Input: part model. Units: mm. Frame: model coordinates. A direction names the side the tool comes from. Coordinates: 2 decimals unless noted, no trailing zeros. Loops run counter-clockwise (first coordinate to the right, second up) from the corner with the lowest first, then second, coordinate; pieces in that order, holes last.
```python
from build123d import *

# Parameters (mm, degrees)
EXTRUDE_1_DEPTH      = 2.5
EXTRUDE_1_DEPTH_BACK = 2.5
SKETCH_2_OUTSIDE_W   = 45.04
SKETCH_2_OUTSIDE_H   = 51.807
SKETCH_2_OUTSIDE_R   = 2
CUT_EXTRUDE_1_DEPTH  = 2.5
CUT_EXTRUDE_1_DRAFT  = -60
FILLET_2_R           = 4
FILLET_3_R           = 9
SKETCH_3_R           = 2
EXTRUDE_2_DEPTH      = 9
SKETCH_4_W           = 26.934408862
SKETCH_4_H           = 1.5
CUT_EXTRUDE_2_DEPTH  = 7
FILLET_4_R           = 0.5


with BuildPart() as part:
    # 草图1 → 凸台-拉伸1 (new, two sides: drawn at the far end of the back side and taken through both)
    with BuildSketch(Plane.XY.offset(-EXTRUDE_1_DEPTH_BACK)):
        Polygon((-1.165769145, -2.5), (-8.342987205, 6.053475407), (-4.512764989, 9.267413455), (1.165769145, 2.5), (138, 2.5), (138, -2.5), align=None)
    extrude(amount=EXTRUDE_1_DEPTH + EXTRUDE_1_DEPTH_BACK)


with BuildPart() as cut_extrude_1_tool:
    # 草图2 outside → 切除-拉伸1 (with draft: the straight prism first)
    with BuildSketch(Plane(origin=(138, 0, 0), x_dir=(0, 0, -1), z_dir=(1, 0, 0))):
        with Locations((0, 3.3835)):
            Rectangle(SKETCH_2_OUTSIDE_W, SKETCH_2_OUTSIDE_H)
        Circle(SKETCH_2_OUTSIDE_R, mode=Mode.SUBTRACT)
    extrude(amount=-CUT_EXTRUDE_1_DEPTH)
    # 切除-拉伸1: the draft: its side faces are tilted about the plane it starts from
    cut_extrude_1_sides = [cut_extrude_1_tool.faces().sort_by_distance(p)[0] for p in [
        (136.75, -22.52, 0),
        (136.75, 3.3835, -22.52),
        (136.75, 29.287, 0),
        (136.75, 3.3835, 22.52),
        (136.75, 0, 2),
    ]]
    draft(cut_extrude_1_sides, Plane(origin=(138, 0, 0), x_dir=(0, 0, -1), z_dir=(1, 0, 0)), CUT_EXTRUDE_1_DRAFT)


with BuildPart() as part_1:
    add(part.part)

    # 切除-拉伸1: cut by cut_extrude_1_tool
    add(cut_extrude_1_tool.part, mode=Mode.SUBTRACT)

    # 圆角2
    fillet_2_edges = [part_1.edges().sort_by_distance(p)[0] for p in [
        (1.165769145, 2.5, 0),
    ]]
    fillet(fillet_2_edges, radius=FILLET_2_R)

    # 圆角3
    fillet_3_edges = [part_1.edges().sort_by_distance(p)[0] for p in [
        (-1.165769145, -2.5, 0),
    ]]
    fillet(fillet_3_edges, radius=FILLET_3_R)

    # 草图3 → 凸台-拉伸2 (add)
    with BuildSketch(Plane(origin=(-6.427876097, 7.660444431, 0), x_dir=(0.7660444431189749, 0.6427876096865432, 0), z_dir=(-0.6427876096865431, 0.7660444431189748, 0))):
        Circle(SKETCH_3_R)
    extrude(amount=EXTRUDE_2_DEPTH)

    # 草图4 → 切除-拉伸2 (cut)
    with BuildSketch(Plane(origin=(-12.212964584, 14.554844419, 0), x_dir=(0.7660444431189747, 0.6427876096865435, 0), z_dir=(-0.6427876096865434, 0.7660444431189746, 0))):
        Rectangle(SKETCH_4_W, SKETCH_4_H)
    extrude(amount=-CUT_EXTRUDE_2_DEPTH, mode=Mode.SUBTRACT)

    # 圆角4
    fillet_4_edges = [part_1.edges().sort_by_distance(p)[0] for p in [
        (-7.959964983, 6.374869212, 0),
    ]]
    fillet(fillet_4_edges, radius=FILLET_4_R - 0.0001)  # a hair under: the kernel refuses the full size


solid = part_1.part
```
Item 1: Contact query for flat-ended pins moving along their axis: P1, Ø2, axis at x = -9, y = 12.5, coming from the -Z side; P2, Ø8, axis at x = -9.5, y = 11, coming from the +Z side. Output: stop coordinate, or through.
Result:
P1: stops at z = -2
P2: stops at z = 2
Item 2: Line query: L1, parallel to Y at x = 43, z = 0.8; L2, parallel to X at y = 1.5, z = 1.4; L3, parallel to X at y = 0.75, z = -1.2. Output: solid intervals per line, ascending.
Result:
L1: y = -2.5 to 2.5
L2: x = -4.52 to 137.97
L3: x = -3.89 to 138
Item 3: Reachability of faces 1 (the face through (69, 2.5, 0)), 2 (the face through (137.86, 1.52, 1.65)), 3 (the face through (-7.735, 9.175, -0.01)) from +Z, -Z, +X, -X, +Y, -Y: full face, straight path, thin tool, end or side. Return the list, or none.
Result:
face 1: +Z, -Z, +X, +Y
face 2: +X
face 3: -X, +Y
Item 4: Section query A-A (x = 63). Output: boundary loops of the cut face in (y, z).
Result:
outline: (-2.5, -2.5) - (2.5, -2.5) - (2.5, 2.5) - (-2.5, 2.5) - close
